For this review, take the finished solid that the model builds, in its own axes (mm). A direction names the side the tool comes from. Coordinates: 2 decimals unless noted, no trailing zeros. Loops run counter-clockwise (first coordinate to the right, second up) from the corner with the lowest first, then second, coordinate; pieces in that order, holes last. Notation, with made-up numbers: M 64.5,20 L 89.5,20 A17 cw 89.5,29 Z; hole C 12.25,-23.75 d8. An arc over 180 degrees is marked long. Write item = value, one per line.
from build123d import *

# Parameters (mm, degrees)
F0_W     = 25.4
F0_H     = 3.175
F0_W_2   = 38.1
F0_R     = 1.7859375
F0_R_2   = 0.5
F1_DEPTH = 3.175


# Not quite as in the source:
# - a length typed as a fraction of an inch, garbled in the dataset ("3 / 203.2 mm" for 3/8 in), is restored


with BuildPart() as f1:
    # F0 (on Front) → F1 (new body)
    with BuildSketch(Plane.XZ):
        with Locations((-54.5774, 62.9375024)):
            Rectangle(F0_W, F0_H)
        with Locations((16.1738, 62.9375024)):
            Rectangle(F0_W_2, F0_H)
        with Locations((86.925, 62.9375024)):
            Rectangle(F0_W, F0_H)
        with Locations((86.925, -24.0574976)):
            Rectangle(F0_W, F0_H)
        with Locations((16.1738, -24.0574976)):
            Rectangle(F0_W_2, F0_H)
        with Locations((-54.5774, -24.0574976)):
            Rectangle(F0_W, F0_H)
        Polygon((-67.2774, 61.1329712169), (-67.2774, -22.4699976), (-41.8774, -22.4699976), (-2.8762, -22.4699976), (35.2238, -22.4699976), (74.225, -22.4699976), (99.625, -22.4699976), (99.625, 61.3500024), (74.225, 61.3500024), (35.2238, 61.3500024), (-2.8762, 61.3500024), (-41.8774, 61.3500024), (-67.2774, 61.3500024), align=None)
        with Locations((-63.3824, 0)):
            Circle(F0_R, mode=Mode.SUBTRACT)
        with Locations((-55.4124, 0)):
            Circle(F0_R, mode=Mode.SUBTRACT)
        with Locations((-47.4424, 0)):
            Circle(F0_R, mode=Mode.SUBTRACT)
        with Locations((-39.4724, 0)):
            Circle(F0_R, mode=Mode.SUBTRACT)
        with Locations((-31.7, 0)):
            Circle(F0_R, mode=Mode.SUBTRACT)
        with Locations((-23.73, 0)):
            Circle(F0_R, mode=Mode.SUBTRACT)
        with Locations((-15.76, 0)):
            Circle(F0_R, mode=Mode.SUBTRACT)
        with Locations((-7.79, 0)):
            Circle(F0_R, mode=Mode.SUBTRACT)
        Circle(F0_R, mode=Mode.SUBTRACT)
        with Locations((7.97, 0)):
            Circle(F0_R, mode=Mode.SUBTRACT)
        with Locations((15.94, 0)):
            Circle(F0_R, mode=Mode.SUBTRACT)
        with Locations((23.91, 0)):
            Circle(F0_R, mode=Mode.SUBTRACT)
        with Locations((31.88, 0)):
            Circle(F0_R, mode=Mode.SUBTRACT)
        with Locations((39.85, 0)):
            Circle(F0_R, mode=Mode.SUBTRACT)
        with Locations((47.82, 0)):
            Circle(F0_R, mode=Mode.SUBTRACT)
        with Locations((55.79, 0)):
            Circle(F0_R, mode=Mode.SUBTRACT)
        with Locations((63.76, 0)):
            Circle(F0_R, mode=Mode.SUBTRACT)
        with Locations((71.73, 0)):
            Circle(F0_R, mode=Mode.SUBTRACT)
        with Locations((79.7, 0)):
            Circle(F0_R, mode=Mode.SUBTRACT)
        with Locations((87.67, 0)):
            Circle(F0_R, mode=Mode.SUBTRACT)
        with Locations((95.64, 0)):
            Circle(F0_R, mode=Mode.SUBTRACT)
        with Locations((-32.93, 40.005)):
            Circle(F0_R_2, mode=Mode.SUBTRACT)
        Polygon((-30.03, 33.705), (-30.03, 46.305), (-18.43, 46.305), (-6.83, 46.305), (-6.83, 33.705), (-18.43, 33.705), align=None, mode=Mode.SUBTRACT)
        with Locations((-3.93, 40.005)):
            Circle(F0_R_2, mode=Mode.SUBTRACT)
    extrude(amount=F1_DEPTH)


solid = f1.part
Q1. Add section D-D (x = 63.76). Write out the cut boundary in (y, z) (3 decimals), and give its area (3 significant figures).
Solved:
outline = M -3.175,-22.47 L 0,-22.47 L 0,-1.786 L -3.175,-1.786 Z; M -3.175,1.786 L 0,1.786 L 0,61.35 L -3.175,61.35 Z
area = 255 mm²
Q2. Add section B-B (x = 31.88). Write out the cut boundary in (y, z) (3 decimals), and give its area (3 significant figures).
Solved:
outline = M -3.175,-25.645 L 0,-25.645 L 0,-1.786 L -3.175,-1.786 Z; M -3.175,1.786 L 0,1.786 L 0,64.525 L -3.175,64.525 Z
area = 275 mm²
Q3. For line 1 along Z through (x, y) = (-7.79, -1.75) (3 decimals); line 2 along Z through (x, y) = (-32.93, -2.1) (3 decimals); line 3 along X through (y, z) = (-0.05, 37.5) (3 decimals), list the stretches that pass through material, from the lowest coordinate up.
Solved:
line_1 = -22.47 to -1.786, 1.786 to 33.705, 46.305 to 61.35
line_2 = -22.47 to -1.295, 1.295 to 39.505, 40.505 to 61.35
line_3 = -67.277 to -30.03, -6.83 to 99.625
Q4. Draft analysis for pull direction Z (two halves, no side actions). For faces 1 (the face through (55, -2, 61.35)), 2 (the face through (-57.197, -1.565, 0.079)), 3 (the face through (-2.876, -2, 63)), state which applies: +Z half, -Z half, draft (parallel to the pull), parting line (faces both ways), or undercut.
Solved:
face_1 = +Z half
face_2 = undercut
face_3 = draft
Q5. For pin 1 Ø1 at (x, y) = (-27.5, -2) entering from +Z; pin 2 Ø1 at (x, y) = (60.5, -1) entering from -Z, all flat-tipped, find the tip position at first contact; note any pin that passes through.
Solved:
pin_1 = 61.35
pin_2 = -22.47
Q6. Add section A-A (x = -15.76). Write out the cut boundary in (y, z) (3 decimals), and give its area (3 significant figures).
Solved:
outline = M -3.175,-22.47 L 0,-22.47 L 0,-1.786 L -3.175,-1.786 Z; M -3.175,1.786 L 0,1.786 L 0,33.705 L -3.175,33.705 Z; M -3.175,46.305 L 0,46.305 L 0,61.35 L -3.175,61.35 Z
area = 215 mm²
Q7. Machinability: for faces 4 (the face through (-2.876, -2, -24)), 5 (the face through (-19, -2, 46.305)), 6 (the face through (35.224, -2, 63)), which of the approach directions +Z, -Z, +X, -X, +Y, -Y give a long, thin tool a straight path to every point of the face, cutting with its end or side? Answer none if there is none.
Solved:
face_4 = -Z, +Y, -Y
face_5 = +Y, -Y
face_6 = +Z, +Y, -Y
Q8. Add section C-C (z = 0). State how many separate pieces and enclosed holes the cut face has, and give its area (3 significant figures).
Solved:
separate_pieces = 22
enclosed_holes = 0
area = 292 mm²
